For this review, take the finished solid that the model builds, in its own axes (mm). Face numbers are marked on the shaded views. A direction names the side the tool comes from. Give positions to 0.01 mm unless a question says otherwise; leave off trailing zeros. Loops run counter-clockwise (first coordinate to the right, second up) from the corner with the lowest first, then second, coordinate; pieces in that order, holes last.
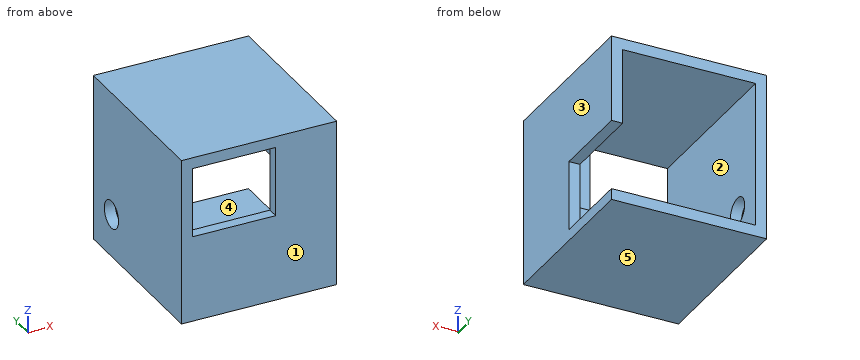
```python
from build123d import *

# Parameters (mm, degrees)
ESQUISSE1_W             = 28
ESQUISSE1_H             = 31
BOSS_EXTRU_1_DEPTH      = 30.2
COQUE1_T                = -2
ENL_V_MAT_EXTRU_1_REACH = 30
ESQUISSE2_W             = 12.6
ESQUISSE2_H             = 15
ENL_V_MAT_EXTRU_2_REACH = 4
ESQUISSE3_W             = 15
ESQUISSE3_H             = 12.6
ESQUISSE4_W             = 24
ESQUISSE4_H             = 12.6
BOSS_EXTRU_2_DEPTH      = 1.5
ENL_V_MAT_EXTRU_4_REACH = 30
ESQUISSE10_R            = 2.5


with BuildPart() as part:
    # Esquisse1 → Boss.-Extru.1 (new body)
    with BuildSketch(Plane.XY):
        with Locations((14, 15.5)):
            Rectangle(ESQUISSE1_W, ESQUISSE1_H)
    extrude(amount=BOSS_EXTRU_1_DEPTH)

    # Coque1
    coque1_openings = [part.faces().sort_by_distance(p)[0] for p in [
        (14, 31, 15.1),
    ]]
    offset(amount=COQUE1_T, openings=coque1_openings, kind=Kind.INTERSECTION)

    # Esquisse2 → Enlèv. mat.-Extru.1 (cut, up to next)
    with BuildSketch(Plane(origin=(28, 0, 0), x_dir=(0, 0, -1), z_dir=(1, 0, 0)), mode=Mode.PRIVATE) as enl_v_mat_extru_1_sk1:
        with Locations((-8.3, 23.5)):
            Rectangle(ESQUISSE2_W, ESQUISSE2_H)
    enl_v_mat_extru_1_tool1 = extrude(enl_v_mat_extru_1_sk1.sketch, amount=-ENL_V_MAT_EXTRU_1_REACH, mode=Mode.PRIVATE) & part.part
    add(enl_v_mat_extru_1_tool1.solids().sort_by_distance((28, 23.5, 8.3))[0], mode=Mode.SUBTRACT)

    # Esquisse3 → Enlèv. mat.-Extru.2 (cut, up to next)
    with BuildSketch(Plane(origin=(0, 2, 0), x_dir=(1, 0, 0), z_dir=(0, 1, 0)), mode=Mode.PRIVATE) as enl_v_mat_extru_2_sk1:
        with Locations((9.5, -21.9)):
            Rectangle(ESQUISSE3_W, ESQUISSE3_H)
    enl_v_mat_extru_2_tool1 = extrude(enl_v_mat_extru_2_sk1.sketch, amount=-ENL_V_MAT_EXTRU_2_REACH, mode=Mode.PRIVATE) & part.part
    add(enl_v_mat_extru_2_tool1.solids().sort_by_distance((9.5, 2, 21.9))[0], mode=Mode.SUBTRACT)

    # Esquisse4 → Boss.-Extru.2 (add)
    with BuildSketch(Plane(origin=(0, 2, 0), x_dir=(1, 0, 0), z_dir=(0, 1, 0))):
        with Locations((14, -8.3)):
            Rectangle(ESQUISSE4_W, ESQUISSE4_H)
    extrude(amount=BOSS_EXTRU_2_DEPTH)

    # Esquisse10 → Enlèv. mat.-Extru.4 (cut, up to next)
    with BuildSketch(Plane.ZY, mode=Mode.PRIVATE) as enl_v_mat_extru_4_sk1:
        with Locations((7.728265811, 24.64)):
            Circle(ESQUISSE10_R)
    enl_v_mat_extru_4_tool1 = extrude(enl_v_mat_extru_4_sk1.sketch, amount=-ENL_V_MAT_EXTRU_4_REACH, mode=Mode.PRIVATE) & part.part
    add(enl_v_mat_extru_4_tool1.solids().sort_by_distance((0, 24.64, 7.728266))[0], mode=Mode.SUBTRACT)


solid = part.part
```
Q1. Consider section D-D on y = 8. Give the boundary of the cut face in (x, z).
Answers:
outline: (0, 0) - (28, 0) - (28, 30.2) - (0, 30.2) - close; hole (2, 2) - (26, 2) - (26, 28.2) - (2, 28.2) - close
Q2. Mouldability with a two-part tool opening along X and no side actions: class the marked faces 1, 2 and 3 as +X half, -X half, draft (parallel to the pull), parting line (faces both ways), or undercut.
Answers:
face 1: draft
face 2: undercut
face 3: +X half
Q3. For pin 1 Ø6.5 at (x, z) = (12.5, 10) entering from +Y; pin 2 Ø12 at (x, y) = (7, 17.5) entering from -Z; pin 3 Ø4.5 at (y, z) = (24.64, 7.73) entering from -X; pin 4 Ø2 at (x, z) = (26.5, 11) entering from +Y, all flat-tipped, find the tip position at first contact; note any pin that passes through.
Answers:
pin 1: stops at y = 3.5
pin 2: stops at z = 0
pin 3: passes through
pin 4: stops at y = 16
Q4. For probe 1 along Z at (x, y) = (18.5, 4.5); probe 2 along X at (y, z) = (25.5, 21); probe 3 along Y at (x, z) = (23, 6), list the stretches that pass through material, from the lowest coordinate up.
Answers:
probe 1: z = 0 to 2, 28.2 to 30.2
probe 2: x = 0 to 2, 26 to 28
probe 3: y = 0 to 3.5
Q5. Consider section C-C on y = 17. Give the boundary of the cut face in (x, z), plus the area to 3 significant figures.
Answers:
outline: (0, 0) - (28, 0) - (28, 2) - (2, 2) - (2, 28.2) - (26, 28.2) - (26, 14.6) - (28, 14.6) - (28, 30.2) - (0, 30.2) - close
area: 192 mm2
Q6. Machinability: for the marked faces 4 and 5, which of the approach directions +Z, -Z, +X, -X, +Y, -Y give a long, thin tool a straight path to every point of the face, cutting with its end or side? Answer none if there is none.
Answers:
face 4: +Y
face 5: -Z, +X, -X, +Y, -Y
Q7. Consider section A-A on x = 3.75. Give the boundary of the cut face in (y, z).
Answers:
outline: (0, 0) - (31, 0) - (31, 2) - (3.5, 2) - (3.5, 14.6) - (2, 14.6) - (2, 15.6) - (0, 15.6) - close; (0, 28.2) - (31, 28.2) - (31, 30.2) - (0, 30.2) - close
Q8. Consider section B-B on y = 24.64. Give the boundary of the cut face in (x, z), plus the area to 3 significant figures.
Answers:
outline: (0, 0) - (28, 0) - (28, 2) - (2, 2) - (2, 5.23) - (0, 5.23) - close; (0, 10.23) - (2, 10.23) - (2, 28.2) - (26, 28.2) - (26, 14.6) - (28, 14.6) - (28, 30.2) - (0, 30.2) - close
area: 182 mm2
